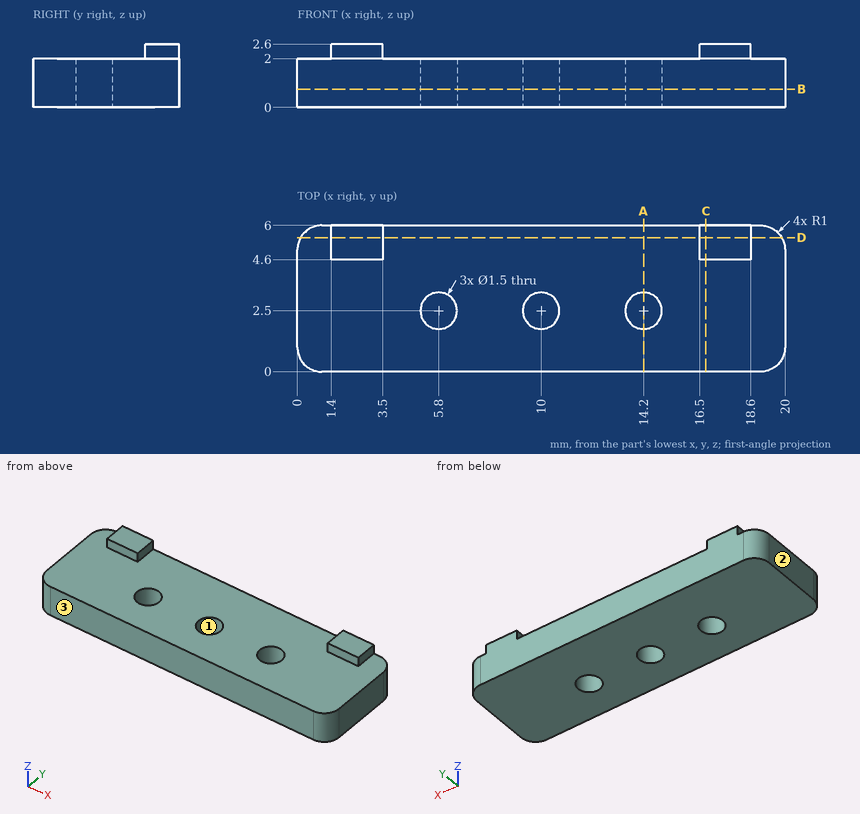
Study the drawing (mm; zero at the part's minimum x, y, z) and answer. Coordinates: 2 decimals unless noted, no trailing zeros. Order: outer loops, then holes, each group sorted by start corner. A loop starts at its lowest first (then second) coordinate and runs counter-clockwise, first axis right, second up. Notation, with made-up numbers: M -11,52.5 L 43,52.5 A5 ccw 43,56.5 Z; hole C 88,-13 d11. An arc over 180 degrees is marked long. Use CSV: the item, a comma, the result in double quotes.
Q1. Section D-D (y = 5.5) is taken. Determine the outline of the cut face in (x, z), then the cut area to 3 significant figures.
Here are the results:
outline,"M 0.13,0 L 19.87,0 L 19.87,2 L 18.6,2 L 18.6,2.6 L 16.5,2.6 L 16.5,2 L 3.5,2 L 3.5,2.6 L 1.4,2.6 L 1.4,2 L 0.13,2 Z"
area,"42.0 mm2"
Q2. Determine the mould class of the marked faces 1, 2 and 3 for opening direction Y: pulls with the +Y half, pulls with the -Y half, needs draft (parallel to the pull), parting line crosses it, or undercut.
Here are the results:
face 1,"undercut"
face 2,"needs draft"
face 3,"pulls with the -Y half"
Q3. Given pin 1 Ø0.7 at (y, z) = (5, 2.5) entering from -X; pin 2 Ø3 at (x, y) = (3, 1.5) entering from +Z; pin 3 Ø0.5 at (x, z) = (3, 2.5) entering from -Y, each flat-ended and moving along its own axis, determine where each tip first touches the part or whether it passes through.
Here are the results:
pin 1,"x = 1.4"
pin 2,"z = 2"
pin 3,"y = 4.6"
Q4. Section A-A (x = 14.2) is taken. Determine the outline of the cut face in (y, z).
Here are the results:
outline,"M 0,0 L 1.75,0 L 1.75,2 L 0,2 Z; M 3.25,0 L 6,0 L 6,2 L 3.25,2 Z"
Q5. Straight lines are drawn through the part: L1, parallel to Y at x = 10, z = 1.5; L2, parallel to X at y = 3.15, z = 1.95; L3, parallel to X at y = 5.1, z = 2.4. For each, find the intervals that lie inside material, in ascending order.
Here are the results:
L1,"0 to 1.75, 3.25 to 6"
L2,"0 to 5.43, 6.17 to 9.63, 10.37 to 13.83, 14.57 to 20"
L3,"1.4 to 3.5, 16.5 to 18.6"
Q6. Section B-B (z = 0.75) is taken. Determine the outline of the cut face in (x, y), then the cut area to 3 significant figures.
Here are the results:
outline,"M 0,1 A1 ccw 1,0 L 19,0 A1 ccw 20,1 L 20,5 A1 ccw 19,6 L 1,6 A1 ccw 0,5 Z; hole C 5.8,2.5 d1.5; hole C 10,2.5 d1.5; hole C 14.2,2.5 d1.5"
area,"114 mm2"
Q7. Section C-C (x = 16.75) is taken. Determine the outline of the cut face in (y, z).
Here are the results:
outline,"M 0,0 L 6,0 L 6,2.6 L 4.6,2.6 L 4.6,2 L 0,2 Z"
